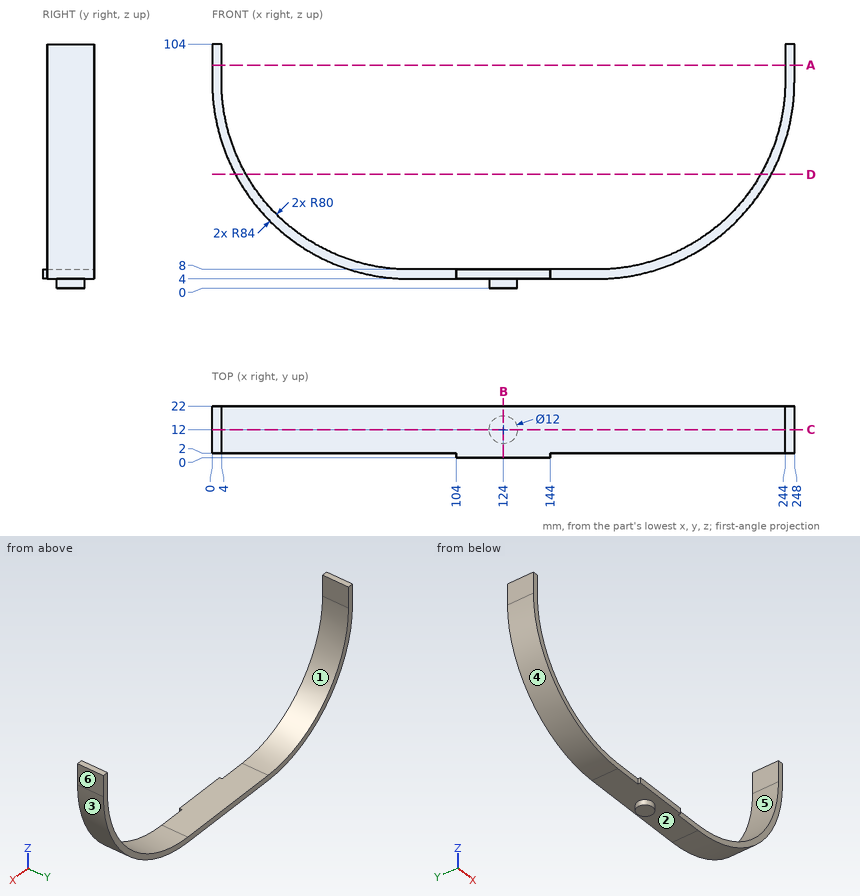
For this review, use the dimensioned drawing (mm, ordinates from the lowest corner) and the shaded views. A direction names the side the tool comes from. Round coordinates to 2 decimals unless told otherwise and drop trailing zeros. Order: outer loops, then holes, each group sorted by start corner. A loop starts at its lowest first (then second) coordinate and runs counter-clockwise, first axis right, second up. Notation, with made-up numbers: M 40.5,10 L 47.5,10 A10 ccw 47.5,17 Z; hole C -13,-39.5 d8. An arc over 180 degrees is marked long. Use a Markdown table: item, result. Add a question column.
Item 1: Add section C-C, the plane y = 12. Give the boundary of the cut face in (x, z).
Item 2: Add section B-B, the plane x = 124. Give the boundary of the cut face in (y, z).
Item 3: Tool access review of the marked faces 5 and 6: name each direction out of +Z, -Z, +X, -X, +Y, -Y from which nothing blocks a thin tool from reaching the whole face with its end or side.
Item 4: Add section D-D, the plane z = 48.5. Give the boundary of the cut face in (x, y), then the cut area to 3 significant figures.
Item 5: Mouldability with a two-part tool opening along X and no side actions: class the marked faces 1, 2, 3 and 4 as released by +X, released by -X, zero draft, split by the parting line, or undercut.
Item 6: To check wall thickness, follow line 1 along X through (y, z) = (11.25, 97); line 2 along Z through (x, y) = (153.5, 19.75); line 3 along X through (y, z) = (18.5, 67). State the ranges of each line that lie inside material, in increasing order.
Item 7: Insertion check: pin 1 (6.5 mm diameter, centred on x = 127.5, y = 15, fed in from +Z); pin 2 (8 mm diameter, centred on x = 86.5, y = 4.5, fed in from -Z); pin 3 (5 mm diameter, centred on y = 6.5, z = 40.5, fed in from +X). Each pin has a flat end and moves straight along its axis. Give the tip position at first contact, or say it passes through.
Item 8: Add section A-A, the plane z = 95. Give the boundary of the cut face in (x, y), then the cut area to 3 significant figures.
Geometry results:
| question | item | result |
|---|---|---|
| 1 | outline | M 0,88 A84 ccw 84,4 L 118,4 L 118,0 L 130,0 L 130,4 L 164,4 A84 ccw 248,88 L 248,104 L 244,104 L 244,88 A80 cw 164,8 L 84,8 A80 cw 4,88 L 4,104 L 0,104 Z |
| 2 | outline | M 0,4 L 6,4 L 6,0 L 18,0 L 18,4 L 22,4 L 22,8 L 0,8 Z |
| 3 | face 5 | +Z, +Y, -Y |
| 3 | face 6 | +Z, -Z, +X, +Y, -Y |
| 4 | outline | M 9.87,2 L 14.43,2 L 14.43,22 L 9.87,22 Z; M 233.57,2 L 238.13,2 L 238.13,22 L 233.57,22 Z |
| 4 | area | 183 mm² |
| 5 | face 1 | undercut |
| 5 | face 2 | zero draft |
| 5 | face 3 | released by +X |
| 5 | face 4 | released by -X |
| 6 | line 1 | x = 0 to 4, 244 to 248 |
| 6 | line 2 | z = 4 to 8 |
| 6 | line 3 | x = 2.67 to 6.81, 241.19 to 245.33 |
| 7 | pin 1 | stops at z = 8 |
| 7 | pin 2 | stops at z = 4 |
| 7 | pin 3 | stops at x = 234.93 |
| 8 | outline | M 0,2 L 4,2 L 4,22 L 0,22 Z; M 244,2 L 248,2 L 248,22 L 244,22 Z |
| 8 | area | 160 mm² |
